For this review, take the finished solid that the model builds, in its own axes (mm). Give positions to 0.01 mm unless a question says otherwise; leave off trailing zeros. Loops run counter-clockwise (first coordinate to the right, second up) from the corner with the lowest first, then second, coordinate; pieces in that order, holes last. Notation, with made-up numbers: (-34.75, 59.25) -> (2.25, 59.25) arc R10 cw to (2.25, 66.25) -> close; hole circle Ø6 at (-38, -10). An arc over 180 degrees is marked (long way). Answer as CSV lines item,"result". Start each with the question number.
Item 1: Clearance check with flat-ended pins moving along their axes: P1, Ø22, axis at x = 4.5, z = -15, coming from the +Y side; P2, Ø1.5, axis at y = 6, z = 15, coming from the -X side; P3, Ø4, axis at x = -1.5, y = 22.5, coming from the -Z side; P4, Ø12, axis at x = -14.5, y = 61.5, coming from the -Z side. State where each tip first meets the part, or that it passes through.
Item 2: Add section B-B on y = 4. State the section outline as (x, z) points, plus the area to 3 significant figures.
Item 3: Add section C-C on y = 59.4. State the section outline as (x, z) points.
Item 4: For L1, parallel to Z at x = 0, y = 26; L2, parallel to X at y = 71, z = 0, list the stretches that pass through material, from the lowest coordinate up. Write a range as from..to.
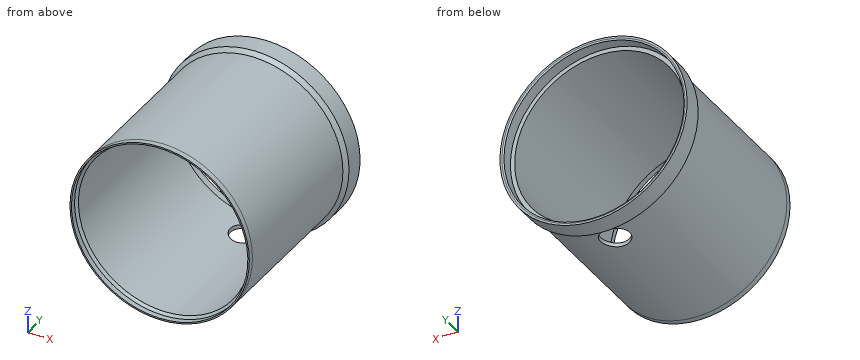
```python
from build123d import *
from build123d.topology import SkipClean

# Parameters (mm, degrees)
SKETCH1_R                = 36.8
SKETCH1_R_2              = 35.2
BOSS_EXTRUDE1_DEPTH      = 70
BOSS_EXTRUDE2_DEPTH      = 5
BOSS_EXTRUDE2_DEPTH_BACK = 5
SKETCH2_R                = 38.4
SKETCH2_R_2              = 36.8
CHAMFER1_SIZE            = 2
FILLET1_R                = 0.8
BOSS_EXTRUDE3_START      = 2.3
SKETCH3_R                = 36.8
SKETCH3_R_2              = 36.2
BOSS_EXTRUDE3_DEPTH      = 2.3
CHAMFER2_SIZE            = 1
SKETCH5_R                = 36.95
CUT_EXTRUDE1_DEPTH       = 10
SKETCH6_R                = 6
CUT_EXTRUDE2_DEPTH       = 10


# Some blends are built 0.0001 mm under size
with BuildPart() as part:
    # Sketch1 → Boss-Extrude1 (new body)
    with BuildSketch(Plane(origin=(0, 0, 0), x_dir=(1, 0, 0), z_dir=(0, 1, 0))):
        with Locations(Location((0, 0, 0), (0, 0, 270))):
            Circle(SKETCH1_R)
        with Locations(Location((0, 0, 0), (0, 0, 270))):
            Circle(SKETCH1_R_2, mode=Mode.SUBTRACT)
    extrude(amount=BOSS_EXTRUDE1_DEPTH)

    # Sketch2 → Boss-Extrude2 (add, two sides: drawn at the far end of the back side and taken through both)
    with BuildSketch(Plane(origin=(0, 70, 0), x_dir=(1, 0, 0), z_dir=(0, 1, 0)).offset(-BOSS_EXTRUDE2_DEPTH_BACK)):
        with Locations(Location((0, 0, 0), (0, 0, 270))):
            Circle(SKETCH2_R)
        with Locations(Location((0, 0, 0), (0, 0, 270))):
            Circle(SKETCH2_R_2, mode=Mode.SUBTRACT)
    extrude(amount=BOSS_EXTRUDE2_DEPTH + BOSS_EXTRUDE2_DEPTH_BACK)

    # Chamfer1
    # the kernel refuses this chamfer: 2 mm, written as the material it takes off along each edge
    with BuildSketch(Plane(origin=(0, 65, 0), x_dir=(0, 0, 1), z_dir=(-1, 0, 0))) as chamfer1_piece_1_section:
        Polygon((38.4 - CHAMFER1_SIZE, 0), (38.4, CHAMFER1_SIZE), (38.4, 0), align=None)
    chamfer1_piece_1 = revolve(axis=Axis((0, 65, 0), (0, 1, 0)), mode=Mode.PRIVATE)
    chamfer1_piece_1 = chamfer1_piece_1 - Plane(origin=(0, 66.172330508, 0), x_dir=(0, 0, 1), z_dir=(0, -1, 0)) * Cylinder(36.8, 154, mode=Mode.PRIVATE)
    add(chamfer1_piece_1, mode=Mode.SUBTRACT)

    # Fillet1
    fillet1_edges = [part.edges().sort_by_distance(p)[0] for p in [
        (0, 75, -36.8),
    ]]
    fillet(fillet1_edges, radius=FILLET1_R)

    # Sketch3 → Boss-Extrude3 (add)
    with BuildSketch(Plane.XZ.offset(BOSS_EXTRUDE3_START)):
        with Locations(Location((0, 0, 0), (0, 0, 270))):
            Circle(SKETCH3_R)
        with Locations(Location((0, 0, 0), (0, 0, 270))):
            Circle(SKETCH3_R_2, mode=Mode.SUBTRACT)
    extrude(amount=-BOSS_EXTRUDE3_DEPTH)

    # Chamfer2
    chamfer2_edges = [part.edges().sort_by_distance(p)[0] for p in [
        (0, 0, -35.2),
    ]]
    chamfer(chamfer2_edges, length=CHAMFER2_SIZE - 0.0001)  # a hair under: the kernel refuses the full size

    # Sketch5 → Cut-Extrude1 (cut)
    with BuildSketch(Plane(origin=(0, 70, 0), x_dir=(1, 0, 0), z_dir=(0, 1, 0))):
        with Locations(Location((0, 0, 0), (0, 0, 270))):
            Circle(SKETCH5_R)
    extrude(amount=CUT_EXTRUDE1_DEPTH, mode=Mode.SUBTRACT)

    # Sketch6 → Cut-Extrude2 (cut)
    with SkipClean():  # the faces are left unmerged after this step: merging them gives an invalid solid
        with BuildSketch(Plane(origin=(0, 0, -36.8), x_dir=(-1, 0, 0), z_dir=(0, 0, -1))):
            with Locations(Location((0, 59.4, 0), (0, 0, 90))):
                Circle(SKETCH6_R)
        extrude(amount=-CUT_EXTRUDE2_DEPTH, mode=Mode.SUBTRACT)


solid = part.part
```
Computed values:
1,P1,"through"
1,P2,"x = -33.93"
1,P3,"z = -36.8"
1,P4,"z = -36.44"
2,outline,"circle Ø73.6 at (0, 0); hole circle Ø70.4 at (0, 0)"
2,area,"362 mm²"
3,outline,"(-6, -36.31) -> (-6, -34.68) arc R35.2 cw (long way) to (6, -34.68) -> (6, -36.31) arc R36.8 ccw (long way) to start"
4,L1,"-36.8..-35.2, 35.2..36.8"
4,L2,"-38.4..-36.95, 36.95..38.4"
